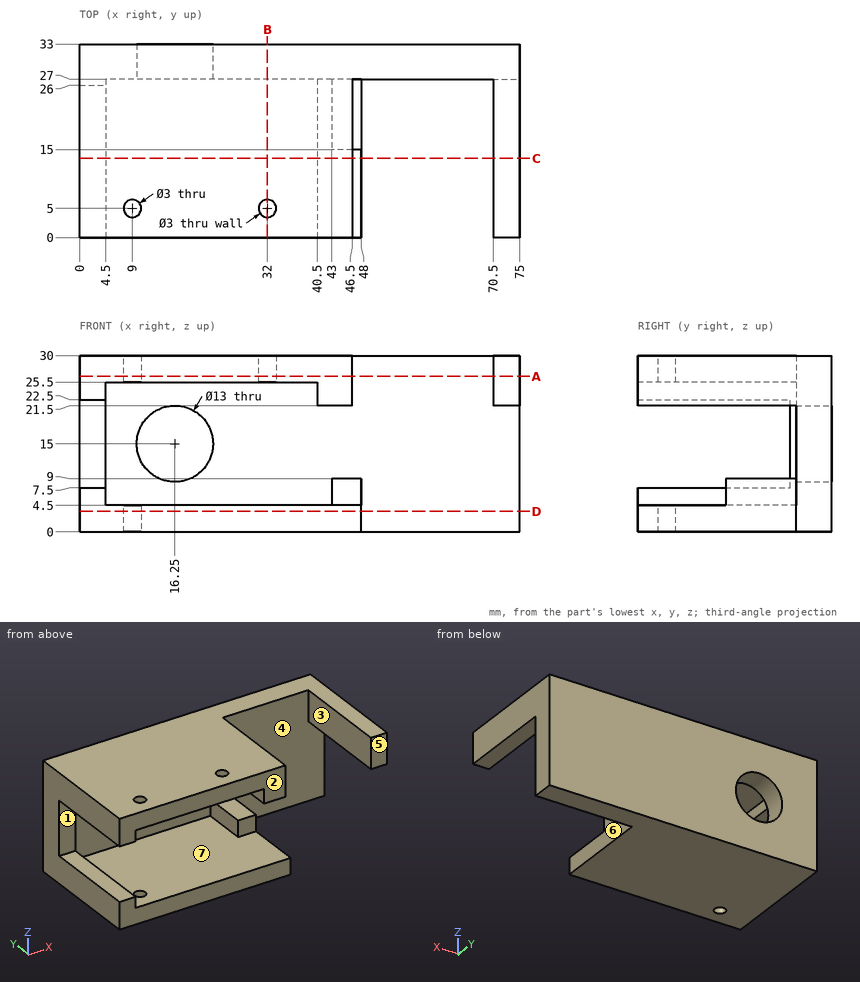
For this review, use the dimensioned drawing (mm, ordinates from the lowest corner) and the shaded views. A direction names the side the tool comes from. Round coordinates to 2 decimals unless told otherwise and drop trailing zeros. Write each loop counter-clockwise with the first axis right and the second up, starting at its lowest first coordinate (ties: lowest second). Pieces come first, ordered by that corner, then holes. Notation, with made-up numbers: (-38, 66.5) -> (-25, 66.5) arc R20 ccw to (-25, 82.5) -> close; hole circle Ø9 at (36, 65). An arc over 180 degrees is marked (long way). One line per item, written item: value. Start each with the question number.
Q1. The part is to be moulded in two halves that separate along X. For the marked faces 5, 6 and 7, say which applies: pulls with the +X half, pulls with the -X half, needs draft (parallel to the pull), parting line crosses it, or undercut.
Q2. Add section A-A (z = 26.5). Give the boundary of the cut face in (x, y).
Q3. Tool access review of the marked faces 1, 2, 3 and 4: name each direction out of +Z, -Z, +X, -X, +Y, -Y from which nothing blocks a thin tool from reaching the whole face with its end or side.
Q4. Add section D-D (z = 3.5). Give the boundary of the cut face in (x, y), then the cut area to 3 significant figures.
Q5. To check wall thickness, follow probe 1 along X at (y, z) = (4.5, 24.75); probe 2 along X at (y, z) = (22, 26.5); probe 3 along Z at (x, y) = (22, 11.5). State the ranges of each line that lie inside material, in increasing order.
Q6. Add section B-B (x = 32). Give the boundary of the cut face in (y, z).
Q7. Insertion check: P1, Ø3, axis at x = 56.5, z = 14, coming from the -Y side; P2, Ø1.3, axis at x = 72, y = 20, coming from the -Z side; P3, Ø2.5, axis at y = 18, z = 5, coming from the +X side. Each pin has a flat end and moves straight along its axis. Give the tip position at first contact, or say it passes through.
Q8. Add section C-C (y = 13.5). Give the boundary of the cut face in (x, z).
Response:
1. face 5: needs draft
1. face 6: pulls with the +X half
1. face 7: undercut
2. outline: (0, 0) -> (46.5, 0) -> (46.5, 27) -> (70.5, 27) -> (70.5, 0) -> (75, 0) -> (75, 33) -> (0, 33) -> close; hole circle Ø3 at (9, 5); hole circle Ø3 at (32, 5)
3. face 1: -X, -Y
3. face 2: +Z, -Z, +X, -X, -Y
3. face 3: +Z, -Z, -Y
3. face 4: -Y
4. outline: (0, 0) -> (48, 0) -> (48, 27) -> (75, 27) -> (75, 33) -> (0, 33) -> close; hole circle Ø3 at (9, 5)
4. area: 1,740 mm^2
5. probe 1: x = 0 to 4.5, 40.5 to 46.5, 70.5 to 75
5. probe 2: x = 0 to 46.5, 70.5 to 75
5. probe 3: z = 0 to 4.5, 25.5 to 30
6. outline: (0, 0) -> (33, 0) -> (33, 30) -> (6.5, 30) -> (6.5, 25.5) -> (27, 25.5) -> (27, 4.5) -> (0, 4.5) -> close; (0, 25.5) -> (3.5, 25.5) -> (3.5, 30) -> (0, 30) -> close
7. P1: stops at y = 27
7. P2: stops at z = 21.5
7. P3: stops at x = 48
8. outline: (0, 0) -> (48, 0) -> (48, 4.5) -> (4.5, 4.5) -> (4.5, 7.5) -> (0, 7.5) -> close; (0, 22.5) -> (4.5, 22.5) -> (4.5, 25.5) -> (40.5, 25.5) -> (40.5, 21.5) -> (46.5, 21.5) -> (46.5, 30) -> (0, 30) -> close; (70.5, 21.5) -> (75, 21.5) -> (75, 30) -> (70.5, 30) -> close
